Input: part model. Units: mm. Frame: model coordinates. Give positions to 0.01 mm unless a question says otherwise; leave off trailing zeros. Loops run counter-clockwise (first coordinate to the right, second up) from the corner with the lowest first, then second, coordinate; pieces in that order, holes last. Notation, with made-up numbers: M 86.5,72.25 L 137.5,72.25 A28 ccw 137.5,90.25 Z; hole C 10,50 d3. An arc over 180 degrees is marked long. Return JSON: item names as keys, results as strings. Group by question number.
```python
from build123d import *

# Parameters (mm, degrees)
SKETCH1_W           = 70
SKETCH1_H           = 70
SKETCH1_R           = 1.5
BOSS_EXTRUDE1_DEPTH = 3
FILLET1_R           = 2
CUT_EXTRUDE1_DEPTH  = 4


with BuildPart() as part:
    # Sketch1 → Boss-Extrude1 (new body)
    with BuildSketch(Plane(origin=(0, 0, 0), x_dir=(1, 0, 0), z_dir=(0, 1, 0))):
        Rectangle(SKETCH1_W, SKETCH1_H)
        with Locations((-32.5, 32.5)):
            Circle(SKETCH1_R, mode=Mode.SUBTRACT)
        with Locations((32.5, 32.5)):
            Circle(SKETCH1_R, mode=Mode.SUBTRACT)
        with Locations((32.5, -32.5)):
            Circle(SKETCH1_R, mode=Mode.SUBTRACT)
        with Locations((-32.5, -32.5)):
            Circle(SKETCH1_R, mode=Mode.SUBTRACT)
    extrude(amount=BOSS_EXTRUDE1_DEPTH)

    # Fillet1
    fillet1_edges = [part.edges().sort_by_distance(p)[0] for p in [
        (35, 1.5, 35),
        (-35, 1.5, 35),
        (-35, 1.5, -35),
        (35, 1.5, -35),
    ]]
    fillet(fillet1_edges, radius=FILLET1_R)

    # Sketch2 → Cut-Extrude1 (cut, through all)
    with BuildSketch(Plane(origin=(0, 3, 0), x_dir=(1, 0, 0), z_dir=(0, 1, 0))):
        with BuildLine():
            Line((30, -32.5), (-30, -32.5))
            ThreePointArc((-30, -32.5), (-30.732233047, -30.732233047), (-32.5, -30))
            Line((-32.5, -30), (-32.5, 30))
            ThreePointArc((-32.5, 30), (-30.732233047, 30.732233047), (-30, 32.5))
            Line((-30, 32.5), (30, 32.5))
            ThreePointArc((30, 32.5), (30.732233047, 30.732233047), (32.5, 30))
            Line((32.5, 30), (32.5, -30))
            ThreePointArc((32.5, -30), (30.732233047, -30.732233047), (30, -32.5))
        make_face()
    extrude(amount=-CUT_EXTRUDE1_DEPTH, mode=Mode.SUBTRACT)


solid = part.part
```
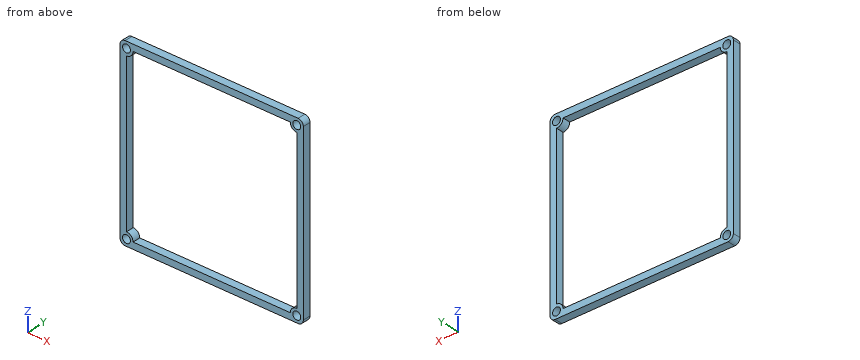
Item 1: Section B-B, the plane x = 25.5. Return loops of the section in (y, z), then the cut area to 3 significant figures.
Item 2: Material intervals for line 1 (Z direction, x = -20, y = 2.3), sorted ascending. Write a range as from..to.
Item 3: Section A-A, the plane y = 0.9. Return loops of the section in (x, z).
Item 4: Section C-C, the plane z = -25.5. Return loops of the section in (x, y), then the cut area to 3 significant figures.
Answer below:
{
 "1": {"outline": "M 0,-35 L 3,-35 L 3,-32.5 L 0,-32.5 Z; M 0,32.5 L 3,32.5 L 3,35 L 0,35 Z", "area": "15.0 mm^2"},
 "2": {"line 1": "-35..-32.5, 32.5..35"},
 "3": {"outline": "M -35,-33 A2 ccw -33,-35 L 33,-35 A2 ccw 35,-33 L 35,33 A2 ccw 33,35 L -33,35 A2 ccw -35,33 Z; hole C -32.5,-32.5 d3; hole C -32.5,32.5 d3; hole M -32.5,-30 A2.5 cw -30,-32.5 L 30,-32.5 A2.5 cw 32.5,-30 L 32.5,30 A2.5 cw 30,32.5 L -30,32.5 A2.5 cw -32.5,30 Z; hole C 32.5,-32.5 d3; hole C 32.5,32.5 d3"},
 "4": {"outline": "M -35,0 L -32.5,0 L -32.5,3 L -35,3 Z; M 32.5,0 L 35,0 L 35,3 L 32.5,3 Z", "area": "15.0 mm^2"}
}
